Check sheet for the drawn part. Datum: minimum x, y, z corner. Units: mm. Round coordinates to 2 decimals unless told otherwise and drop trailing zeros. Write each loop counter-clockwise with the first axis right and the second up, starting at its lowest first coordinate (ties: lowest second). Pieces come first, ordered by that corner, then holes. Notation, with made-up numbers: M 38.25,56.5 L 49.25,56.5 A12 cw 49.25,60.5 Z; hole C 71.25,-4.75 d4. An arc over 180 degrees is marked long. One line per item, written item: value. Start each with the question number.
1. Section check A-A (x = 39.37). Record the boundary of the cut face in (y, z).
2. Section check C-C (y = 2.5). Record the boundary of the cut face in (x, z).
3. Scan lines: probe 1 along Y at (x, z) = (6.35, 9.5); probe 2 along X at (y, z) = (3, 9.5); probe 3 along X at (y, z) = (2.25, 8). Record each from-to range of solid material in increasing order. Write a range as [from, to].
4. Depth check by flat-ended pin: P1, Ø2, axis at x = 37.5, z = 8, coming from the -Y side. Enter the tip coordinate at first touch or a pass-through.
5. Section check B-B (z = 5.25). Count the separate pieces of the cut face and the enclosed holes in it, and give its area (3 significant figures).
6. Release check for a two-part mould opening along X. For the marked faces 1, 2, 3 and 4 record: pulls with the +X half, pulls with the -X half, needs draft (parallel to the pull), parting line crosses it, or undercut.
7. Section check D-D (y = 5.75). Record the boundary of the cut face in (x, z).
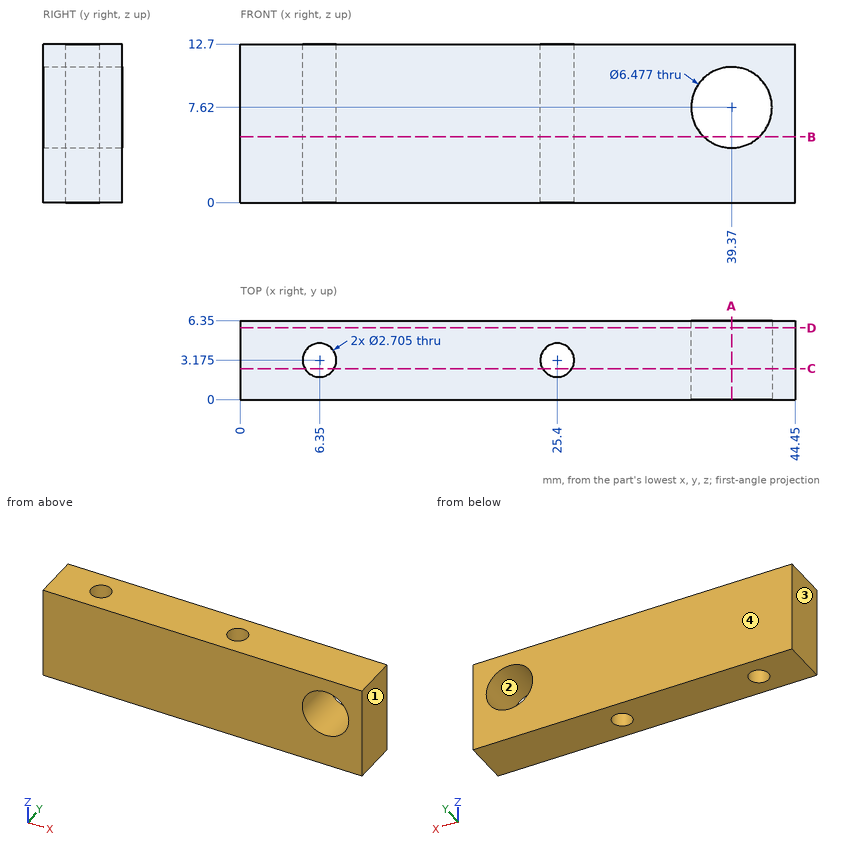
Result sheet:
1. outline: M 0,0 L 6.35,0 L 6.35,4.38 L 0,4.38 Z; M 0,10.86 L 6.35,10.86 L 6.35,12.7 L 0,12.7 Z
2. outline: M 0,0 L 5.18,0 L 5.18,12.7 L 0,12.7 Z; M 7.52,0 L 24.23,0 L 24.23,12.7 L 7.52,12.7 Z; M 26.57,0 L 44.45,0 L 44.45,12.7 L 26.57,12.7 Z; hole C 39.37,7.62 d6.48
3. probe 1: y = [0, 1.82], [4.53, 6.35]
3. probe 2: x = [0, 5.01], [7.69, 24.06], [26.74, 36.73], [42.01, 44.45]
3. probe 3: x = [0, 5.36], [7.34, 24.41], [26.39, 36.15], [42.59, 44.45]
4. P1: passes through
5. separate pieces: 2
5. enclosed holes: 2
5. area: 243 mm2
6. face 1: pulls with the +X half
6. face 2: undercut
6. face 3: pulls with the -X half
6. face 4: needs draft
7. outline: M 0,0 L 44.45,0 L 44.45,12.7 L 0,12.7 Z; hole C 39.37,7.62 d6.48
